Here's how the part is built. I have some questions about the finished solid (model axes, mm). A direction names the side the tool comes from. Round coordinates to 2 decimals unless told otherwise and drop trailing zeros. Order: outer loops, then holes, each group sorted by start corner. A loop starts at its lowest first (then second) coordinate and runs counter-clockwise, first axis right, second up. Notation, with made-up numbers: (26, -9.5) - (78, -9.5) arc R23 cw to (78, 29.5) - close; hole circle Ø7 at (45, 64). An arc over 180 degrees is marked (long way). One line per item, written item: value.
Autodesk Inventor part; units mm, degrees
ref_plane "YZ Plane" through (0, 0, 0) normal (1, 0, 0) x (0, 1, 0)
ref_plane "XZ Plane" through (0, 0, 0) normal (0, 1, 0) x (-1, 0, 0)
ref_plane "XY Plane" through (0, 0, 0) normal (0, 0, 1) x (1, 0, 0)
sketch "Sketch1" plane through (0, 0, 0) normal (0, 0, 1) x (1, 0, 0)
  circle A0 centre (0, 0) radius 50
  dimension "d0" = 100
extrude "Extrusion1" add sketch "Sketch1" along normal blind 10
sketch "Sketch2" plane through (0, 0, 10) normal (0, 0, 1) x (1, 0, 0)
  circle A0 centre (0, 0) radius 40
  dimension "d3" = 80
extrude "Extrusion2" add sketch "Sketch2" along normal blind 15
fillet "Fillet1" radius 3 1 edges at (-50, 0, 10)
sketch "Sketch3" plane through (0, 0, 0) normal (0, 0, -1) x (-1, 0, 0)
  point P0 (0, 0)
  point P1 (0, 0)
hole "Hole1" at (0, 0, 0) direction (0, 0, 1) diameter 20 end through all
fillet "Fillet2" radius 2 1 edges at (-50, 0, 0)
sketch "Sketch5" plane through (0, 0, 0) normal (0, 0, -1) x (-1, 0, 0)
  circle A0 centre (0, 0) radius 10
  line L0 (-2, 12) -> (2, 12)
  line L1 (2, 12) -> (2, 8)
  line L2 (2, 8) -> (-2, 8)
  line L3 (-2, 8) -> (-2, 12)
  point P0 (-2, 10)
  point P1 (-2, 9.798)
  point P2 (2, 9.798)
  dimension "d19" = 4
  dimension "d20" = 4
  dimension "d21" = 2
  dimension "d22" = 12
extrude "Extrusion4" cut sketch "Sketch5" against normal through all contours A0 L3 L0 L1
properties part number "P204" material "Aluminum 6061"
Q1. If we section it at B-B, the plane x = 0: Please give me the cut outline in (y, z), then the cut area to 3 significant figures.
Results list:
outline: (-50, 2) arc R2 ccw to (-48, 0) - (-10, 0) - (-10, 25) - (-40, 25) - (-40, 10) - (-47, 10) arc R3 ccw to (-50, 7) - close; (12, 0) - (48, 0) arc R2 ccw to (50, 2) - (50, 7) arc R3 ccw to (47, 10) - (40, 10) - (40, 25) - (12, 25) - close
area: 1,640 mm²
Q2. We'd pull the mould along X, two halves only. Please class faces 1 (the cylindrical face through (0, -10, 13)), 2 (the cylindrical face through (-8.67, 39.05, 17.4)), 3 (the flat face through (-25, 32, 10)): released by +X, released by -X, zero draft, split by the parting line, or undercut.
Results list:
face 1: undercut
face 2: split by the parting line
face 3: zero draft
Q3. If we section it at A-A, the plane y = 0: Please give me the cut outline in (x, z).
Results list:
outline: (-50, 2) arc R2 ccw to (-48, 0) - (-10, 0) - (-10, 25) - (-40, 25) - (-40, 10) - (-47, 10) arc R3 ccw to (-50, 7) - close; (10, 0) - (48, 0) arc R2 ccw to (50, 2) - (50, 7) arc R3 ccw to (47, 10) - (40, 10) - (40, 25) - (10, 25) - close
Q4. If we section it at C-C, the plane z = 17.25: Please give me the cut outline in (x, y), then the cut area to 3 significant figures.
Results list:
outline: circle Ø80 at (0, 0); hole (-2, 9.8) arc R10 ccw (long way) to (2, 9.8) - (2, 12) - (-2, 12) - close
area: 4,700 mm²
Q5. If I drill on line 1 along Y through (x, z) = (-0.5, 7); line 2 along Y through (x, z) = (0, 17); line 3 along Z through (x, y) = (-34.5, -21), over which ranges is the centre line in solid material (lowest first)?
Results list:
line 1: -50 to -9.99, 12 to 50
line 2: -40 to -10, 12 to 40
line 3: 0 to 10
Q6. Will these pins go through, and if not, where does the flat tip stop? pin 1 (10 mm diameter, centred on x = 26.5, z = 12.5, fed in from +Y); pin 2 (3 mm diameter, centred on x = 1, z = 12, fed in from -Y); pin 3 (8 mm diameter, centred on x = 30.5, z = 6, fed in from -Y).
Results list:
pin 1: y = 43.68
pin 2: y = -40
pin 3: y = -42.4
Q7. Which directions (+Z, -Z, +X, -X, +Y, -Y) give clear straight access to the entire face, cutting with the end or side of a thin tool? Please do faces 4 (the flat face through (-2, 11, 12)), 5 (the flat face through (8, -8, 25)).
Results list:
face 4: +Z, -Z
face 5: +Z, +X, -X, +Y, -Y
